The model under review builds one solid part; all positions refer to its coordinate system, in mm. Round coordinates to 2 decimals unless told otherwise and drop trailing zeros. Write each loop counter-clockwise with the first axis right and the second up, starting at its lowest first coordinate (ties: lowest second). Pieces come first, ordered by that corner, then holes.
Item 1: To check wall thickness, follow L1, parallel to X at y = 34, z = 1.45; L2, parallel to X at y = 2, z = 1.65; L3, parallel to Y at x = 140, z = -0.45. State the ranges of each line that lie inside material, in increasing order.
Item 2: Clearance check with flat-ended pins moving along their axes: pin 1 Ø1.9 at (x, y) = (118.49, 32.7) entering from +Z; pin 2 Ø5 at (x, y) = (-140, 5) entering from -Z; pin 3 Ø1.5 at (x, z) = (-24, 1) entering from -Y; pin 4 Ø4 at (x, y) = (-118.49, 32.7) entering from +Z. State where each tip first meets the part, or that it passes through.
Item 3: Add section B-B (x = 0). Give the boundary of the cut face in (y, z), plus the area to 3 significant figures.
Item 4: Add section A-A (y = 13). Give the boundary of the cut face in (x, z).
```python
from build123d import *

# Parameters (mm, degrees)
SKETCH_1_R          = 1.6
EXTRUDE_1_DEPTH     = 2.5
CUT_EXTRUDE_2_DEPTH = 156.503987087
CHAMFER_2_SIZE      = 4
SKETCH_6_R          = 1
CUT_EXTRUDE_3_DEPTH = 156.503987087
SKETCH_7_R          = 2.1
SKETCH_7_R_2        = 1.6
CUT_EXTRUDE_4_DEPTH = 156.503987087
CHAMFER_3_SIZE      = 1.5
CHAMFER_4_SIZE      = 2


with BuildPart() as part:
    # 草图1 → 凸台-拉伸1 (new, symmetric)
    with BuildSketch(Plane.XY):
        Polygon((-150, 40.7), (-150, -10), (-130, -10), (-130, 15.7), (130, 15.7), (130, -10), (150, -10), (150, 40.7), align=None)
        with Locations((-140, 5)):
            Circle(SKETCH_1_R, mode=Mode.SUBTRACT)
        with Locations((-140, -5)):
            Circle(SKETCH_1_R, mode=Mode.SUBTRACT)
        with Locations((140, 5)):
            Circle(SKETCH_1_R, mode=Mode.SUBTRACT)
        with Locations((140, -5)):
            Circle(SKETCH_1_R, mode=Mode.SUBTRACT)
    extrude(amount=EXTRUDE_1_DEPTH, both=True)

    # 草图4 → 切除-拉伸2 (cut, through all)
    with BuildSketch(Plane.XY.offset(2.5)):
        Polygon((118, 40.7), (113, 35.7), (-113, 35.7), (-118, 40.7), align=None)
    extrude(amount=-CUT_EXTRUDE_2_DEPTH, mode=Mode.SUBTRACT)

    # 倒角2
    chamfer_2_edges = [part.edges().sort_by_distance(p)[0] for p in [
        (-150, -10, 0),
        (-150, 40.7, 0),
        (150, 40.7, 0),
        (150, -10, 0),
        (130, -10, 0),
        (-130, -10, 0),
    ]]
    chamfer(chamfer_2_edges, length=CHAMFER_2_SIZE)

    # 草图6 → 切除-拉伸3 (cut, through all)
    with BuildSketch(Plane(origin=(0, 0, -2.5), x_dir=(-1, 0, 0), z_dir=(0, 0, -1))):
        with Locations((129, 15.7)):
            Circle(SKETCH_6_R)
        with Locations((-129, 15.7)):
            Circle(SKETCH_6_R)
    extrude(amount=-CUT_EXTRUDE_3_DEPTH, mode=Mode.SUBTRACT)

    # 草图7 → 切除-拉伸4 (cut, through all)
    with BuildSketch(Plane.XY.offset(2.5)):
        with Locations((-138.5, 25.2)):
            Circle(SKETCH_7_R)
        with Locations((118.485281374, 32.7)):
            Circle(SKETCH_7_R_2)
        with Locations((-118.485281374, 32.7)):
            Circle(SKETCH_7_R_2)
        with Locations(Location((138.5, 25.2, 0), (0, 0, 180))):
            Circle(SKETCH_7_R)
    extrude(amount=-CUT_EXTRUDE_4_DEPTH, mode=Mode.SUBTRACT)

    # 倒角3
    chamfer_3_edges = [part.edges().sort_by_distance(p)[0] for p in [
        (116.885281374, 32.7, 2.5),
        (-120.085281374, 32.7, 2.5),
    ]]
    chamfer(chamfer_3_edges, length=CHAMFER_3_SIZE)

    # 倒角4
    chamfer_4_edges = [part.edges().sort_by_distance(p)[0] for p in [
        (-140.6, 25.2, 2.5),
        (140.6, 25.2, 2.5),
    ]]
    chamfer(chamfer_4_edges, length=CHAMFER_4_SIZE)


solid = part.part
```
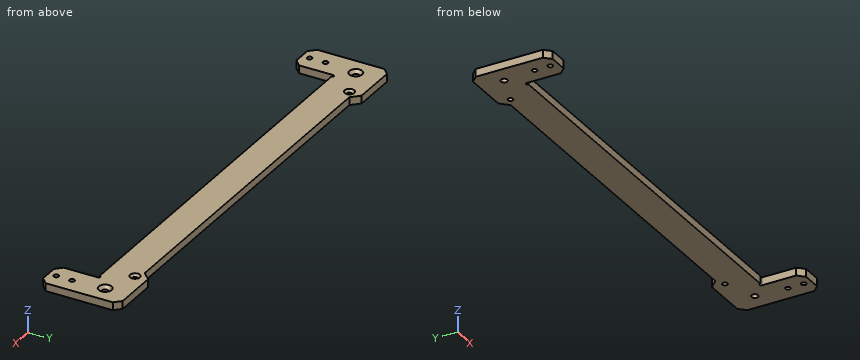
Numbers:
1. L1: x = -150 to -120.07, -116.9 to 116.9, 120.07 to 150
1. L2: x = -150 to -130, 130 to 150
1. L3: y = -10 to -6.6, -3.4 to 3.4, 6.6 to 23.73, 26.67 to 40.7
2. pin 1: passes through
2. pin 2: stops at z = -2.5
2. pin 3: stops at y = 15.7
2. pin 4: stops at z = 1.4
3. outline: (15.7, -2.5) - (35.7, -2.5) - (35.7, 2.5) - (15.7, 2.5) - close
3. area: 100 mm2
4. outline: (-150, -2.5) - (-130, -2.5) - (-130, 2.5) - (-150, 2.5) - close; (130, -2.5) - (150, -2.5) - (150, 2.5) - (130, 2.5) - close
